Source: CAD feature listing. Evaluate the final solid. Frame: model axes, mm. Face numbers are marked on the shaded views. A direction names the side the tool comes from. Give positions to 0.01 mm unless a question says otherwise; leave off trailing zeros. Loops run counter-clockwise (first coordinate to the right, second up) from the corner with the lowest first, then second, coordinate; pieces in that order, holes last. Notation, with made-up numbers: M 49,30 L 101,30 A22 cw 101,39 Z; hole C 89,14.5 d5. An arc over 180 degrees is marked long. Answer in a Markdown table with one row per item.
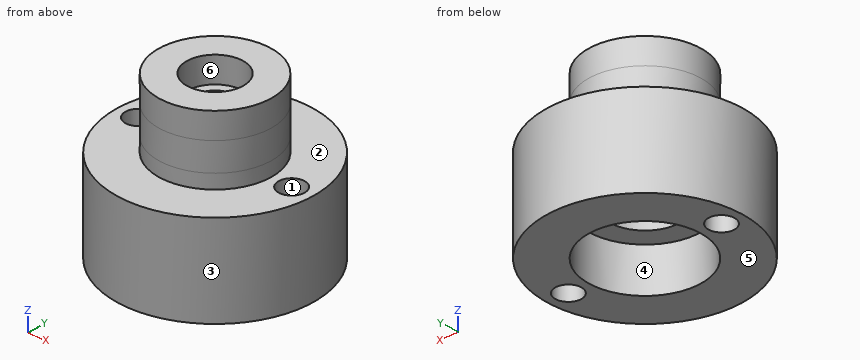
Autodesk Inventor part; units mm, degrees
ref_plane "YZ Plane" through (0, 0, 0) normal (1, 0, 0) x (0, 1, 0)
ref_plane "XZ Plane" through (0, 0, 0) normal (0, 1, 0) x (-1, 0, 0)
ref_plane "XY Plane" through (0, 0, 0) normal (0, 0, 1) x (1, 0, 0)
sketch "Sketch1" plane through (0, 0, 0) normal (0, 0, 1) x (1, 0, 0)
  circle A0 centre (0, 0) radius 4.7625
  circle A1 centre (0, 0) radius 3.175
  dimension "d0" = 6.35
  dimension "d2" = 9.525
extrude "Extrusion1" add sketch "Sketch1" against normal blind 1.5875
sketch "Sketch2" plane through (0, 0, -1.5875) normal (0, 0, -1) x (-1, 0, 0)
  circle A0 centre (0, 0) radius 4.7625
  circle A1 centre (0, 0) radius 6.35
  dimension "d5" = 12.7
extrude "Extrusion2" add sketch "Sketch2" along normal blind 1.5875 contours A0 | A1
sketch "Sketch3" plane through (0, 0, -3.175) normal (0, 0, -1) x (-1, 0, 0)
  circle A0 centre (0, 0) radius 6.35
  circle A1 centre (0, 0) radius 3.9688
  dimension "d9" = 7.9375
extrude "Extrusion3" add sketch "Sketch3" along normal blind 2.54
hole "Hole1" at (0, 0, -3.175) direction (0, 0, 1) diameter 4.318 depth 25.4 tip angle 118
sketch "Sketch4" plane through (0, 0, -5.715) normal (0, 0, -1) x (-1, 0, 0)
  circle A0 centre (0, 0) radius 3.9687
  circle A1 centre (0, 0) radius 6.35
  circle A2 centre (0, 0) radius 11.1125
  dimension "d21" = 22.225
extrude "Extrusion4" add sketch "Sketch4" along normal blind 5.969 contours A1 | A2
sketch "Sketch5" plane through (0, 0, -11.684) normal (0, 0, -1) x (-1, 0, 0)
  circle A0 centre (0, 0) radius 11.1125
  circle A1 centre (0, 0) radius 6.35
  dimension "d25" = 12.7
extrude "Extrusion5" add sketch "Sketch5" along normal blind 4.9784
sketch "Sketch9" plane through (0, 0, -5.715) normal (0, 0, 1) x (1, 0, 0)
  circle A0 centre (0, 0) radius 11.1125
  circle A1 centre (0, 0) radius 6.35
  line L0 (-8.7312, 0) -> (0, 0) construction
  line L1 (0, 0) -> (8.7312, 0) construction
  circle A2 centre (0, 0) radius 8.7312 construction
  dimension "d53" = 2.3813
  dimension "d54" = 2.3813
hole "Hole4" at (-8.7312, 0, -5.715) at (8.7312, 0, -5.715) direction (0, 0, -1) diameter 2.9464 end through all
sketch "Sketch10" plane through (0, 0, -5.715) normal (0, 0, 1) x (1, 0, 0)
  circle A0 centre (-8.7312, 0) radius 1.4732
  circle A1 centre (8.7312, 0) radius 1.4732
  circle A2 centre (0, 0) radius 11.1125
  circle A3 centre (0, 0) radius 6.35
extrude "Extrusion6" add sketch "Sketch10" along normal blind 0.9588
sketch "Sketch11" plane through (0, 0, -1.5875) normal (0, 0, 1) x (1, 0, 0)
  circle A0 centre (0, 0) radius 6.35
  circle A1 centre (0, 0) radius 3.175
extrude "Extrusion7" add sketch "Sketch11" along normal blind 2.8914
sketch "Sketch12" plane through (0, 0, -4.7561) normal (0, 0, 1) x (1, 0, 0)
  circle A0 centre (0, 0) radius 6.35
  circle A1 centre (8.7312, 0) radius 1.4732
  circle A2 centre (-8.7312, 0) radius 1.4732
  circle A3 centre (0, 0) radius 11.1125
extrude "Extrusion8" cut sketch "Sketch12" against normal blind 1.5875
equation "\"d53\" = d54"
equation "\"BendRadius\" = Thickness"
equation "\"BendReliefWidth\" = Thickness"
equation "\"BendReliefDepth\" = 0.5 * Thickness"
equation "\"CornerReliefSize\" = 4 * Thickness"
equation "\"MinimumRemnant\" = 2 * Thickness"
equation "\"TransitionRadius\" = BendRadius"
equation "\"JacobiRadiusSize\" = Thickness"
equation "\"GapSize\" = Thickness"
properties part number "Pneumatic Connector - Bearing Hold" material "Aluminum 6061"
1) Material intervals for L1, parallel to Y at x = 0, z = -0.95 (3 decimals); L2, parallel to Y at x = 0, z = -3.85; L3, parallel to Z at x = -1.5, y = 6, sorted ascending.
Reply:
| item | result |
|---|---|
| L1 | y = -6.35 to -3.175, 3.175 to 6.35 |
| L2 | y = -6.35 to -3.97, 3.97 to 6.35 |
| L3 | z = -11.68 to 1.3 |
2) Pin query (flat end, axial travel): pin 1 Ø3 at (x, z) = (2, -7.5) entering from +Y; pin 2 Ø9 at (x, y) = (0, 0) entering from -Z; pin 3 Ø1.5 at (y, z) = (-1.5, -1.5) entering from +X; pin 4 Ø6.5 at (x, y) = (-0.5, -1) entering from +Z. Return the tip coordinate at first contact, or that it passes through.
Reply:
| item | result |
|---|---|
| pin 1 | stops at y = 11.1 |
| pin 2 | stops at z = -11.68 |
| pin 3 | stops at x = 6.31 |
| pin 4 | stops at z = 1.3 |
3) Section C-C, the plane y = -1. Count the separate pieces of the cut face and the enclosed holes in it, then the cut area to 3 significant figures.
Reply:
| item | result |
|---|---|
| separate pieces | 4 |
| enclosed holes | 0 |
| area | 128 mm² |
4) Pull-direction query (Y, two-part tool) for the marked faces 1, 2 and 3; classes: released by +Y, released by -Y, zero draft, split by the parting line, or undercut.
Reply:
| item | result |
|---|---|
| face 1 | undercut |
| face 2 | zero draft |
| face 3 | split by the parting line |
5) Section B-B, the plane y = 5. Return loops of the section in (x, z), then the cut area to 3 significant figures.
Reply:
| item | result |
|---|---|
| outline | M -9.92,-16.66 L -3.91,-16.66 L -3.91,-11.68 L 3.91,-11.68 L 3.91,-16.66 L 9.92,-16.66 L 9.92,-6.34 L 3.91,-6.34 L 3.91,1.3 L -3.91,1.3 L -3.91,-6.34 L -9.92,-6.34 Z |
| area | 226 mm² |
6) Set-up query: the marked faces 4, 5 and 6. Return all of +Z, -Z, +X, -X, +Y, -Y with unobstructed straight access to the full face (end or side cutting, diameter ignored); none if empty.
Reply:
| item | result |
|---|---|
| face 4 | -Z |
| face 5 | -Z, +X, -X, +Y, -Y |
| face 6 | +Z |
7) Section D-D, the plane z = -9.75. Return loops of the section in (x, y) (1 decimal), then the cut area to 3 significant figures.
Reply:
| item | result |
|---|---|
| outline | C 0,0 d22.2; hole C -8.7,0 d2.9; hole C 0,0 d7.9; hole C 8.7,0 d2.9 |
| area | 325 mm² |
